Autodesk Inventor part; units mm, degrees
ref_plane "Work Plane1" through (8.89, -49.6518, 0) normal (1, 0, 0) x (0, 1, 0)
ref_plane "XZ Plane" through (0, 0, 0) normal (0, 1, 0) x (-1, 0, 0)
ref_plane "XY Plane" through (0, 0, 0) normal (0, 0, 1) x (1, 0, 0)
sketch "Sketch1" plane through (0, 0, 0) normal (0, 0, 1) x (1, 0, 0)
  line L0 (0, 0) -> (4.826, 4.3221)
  line L1 (4.826, 4.3221) -> (10.16, 0)
  line L2 (10.16, 0) -> (11.43, 6.2217)
  line L3 (0, 0) -> (-4.975, 5.229)
  arc A0 (11.43, 6.2217) -> (-4.975, 5.229) centre (5.08, -24.8868) ccw
  circle A1 centre (5.08, -24.8868) radius 25.4 construction
  circle A2 centre (5.08, -24.8868) radius 21.59 construction
  arc A3 (5.08, -47.1118) -> (7.7653, -46.949) centre (5.08, -24.8868) ccw
  circle A4 centre (5.08, -49.6518) radius 1.5875
  line L4 (5.08, -49.6518) -> (5.08, -46.4768) construction
  arc A5 (-14.879, -4.4376) -> (5.08, -53.4618) centre (5.08, -24.8868) ccw
  arc A6 (5.08, -53.4618) -> (7.7653, -46.949) centre (5.08, -49.6518) ccw
  line L5 (0, 0) -> (0, -3.2502)
  line L6 (-4.975, 5.229) -> (-14.879, -4.4376)
  arc A7 (0, -3.2502) -> (5.08, -47.1118) centre (5.08, -24.8868) ccw
  dimension "d40" = 43.18
  dimension "d0" = 31.75
  dimension "d2" = 50.8
  dimension "d3" = 29.21
  dimension "d4" = 30
  dimension "d5" = 10.16
  dimension "d6" = 5.334
  dimension "d42" = 44.45
  dimension "d43" = 3.175
  dimension "d44" = 3.175
  dimension "d47" = 3.81
extrude "Extrusion1" add sketch "Sketch1" along normal blind 6.35 contours L5 A7 A3 A6 A5 L6 L3
ref_plane "Work Plane1" through (8.89, -49.6518, 0) normal (1, 0, 0) x (0, 1, 0)
sketch "Sketch5" plane through (8.89, -49.6518, 0) normal (1, 0, 0) x (0, 1, 0)
  line L0 (-1.5875, 6.35) -> (1.5875, 6.35) construction
  line L1 (1.5875, 0) -> (-1.5875, 0) construction
  line L2 (-3.556, 1.397) -> (3.556, 1.397)
  line L3 (3.556, 1.397) -> (3.556, 4.953)
  line L4 (3.556, 4.953) -> (-3.556, 4.953)
  line L5 (-3.556, 4.953) -> (-3.556, 1.397)
  line L6 (-3.81, 0) -> (-3.81, 6.35) construction
  point P0 (49.6518, 0)
  point P1 (3.556, 3.175)
  point P2 (-3.81, 3.175)
  point P3 (0, 4.953)
  point P4 (0, 6.35)
  dimension "d48" = 3.556
  dimension "d49" = 7.112
extrude "Extrusion5" cut sketch "Sketch5" against normal blind 7.62
fillet "Fillet2" radius 1.27 5 edges at (7.7653, -46.949, 5.6515) (7.7653, -46.949, 0.6985) (0, -3.2502, 3.175) (0, 0, 3.175) (-4.975, 5.229, 3.175)
properties part number "BearingHolder1" material "ABS Plastic"
Input: part model. Units: mm. Frame: model coordinates. A direction names the side the tool comes from. Coordinates: 2 decimals unless noted, no trailing zeros. Loops run counter-clockwise (first coordinate to the right, second up) from the corner with the lowest first, then second, coordinate; pieces in that order, holes last. Notation, with made-up numbers: (-21, 45.25) - (16, 45.25) arc R16 cw to (16, 64.25) - close; hole circle Ø4 at (-11.75, -25.5). An arc over 180 degrees is marked (long way). Answer in a Markdown table with one row per item. Add a question column.
Item 1: Access query for faces 4 (the cylindrical face through (4.74, -48.1, 5.64)), 5 (the cylindrical face through (-0.265, -3.043, 3.219)), 6 (the cylindrical face through (6.108, -47.088, 5.642)), 7 (the flat face through (5.1, -51.4, 4.953)), 8 (the flat face through (0, -1, 3)). Directions: +Z, -Z, +X, -X, +Y, -Y. A direction counts if a zero-diameter tool reaches every point of the face in a straight line with its end or side. Return the directions, or none.
Item 2: Mould query, pull axis X, two halves, no side actions, for faces 1 (the cylindrical face through (7.93, -52.18, 5.25)), 2 (the cylindrical face through (4.74, -48.1, 0.69)), 3 (the flat face through (-17, -31, 6.35)). Classes: released by +X, released by -X, zero draft, split by the parting line, or undercut.
Item 3: Line query: line 1 along Y through (x, z) = (5.08, 5.8); line 2 along Y through (x, z) = (-9.5, 4); line 3 along X through (y, z) = (-49, 5). Output: solid intervals per line, ascending. Write a range as [from, to].
Item 4: Section query A-A on z = 2.25. Return the cut outline in (x, y) (3 decimals), then the cut area to 3 significant figures.
Item 5: Section query D-D on y = -14.5. Return the cut outline in (x, z).
Item 6: Section query C-C on x = -13. Return the cut outline in (y, z).
Item 7: Section query B-B on x = -8. Return the cut outline in (y, z).
Item 8: Contact query for flat-ended pins moving along their axis: P1, Ø5, axis at x = 5.5, y = -51, coming from the -Z side; P2, Ø1.4, axis at y = -1.5, z = 4, coming from the +X side; P3, Ø3, axis at y = -36, z = 3.5, coming from the -X side; P4, Ø1, axis at y = -40, z = 4, coming from the +X side. Output: stop coordinate, or through.
Recorded:
| question | item | result |
|---|---|---|
| 1 | face 4 | +Z, -Z |
| 1 | face 5 | +Z, -Z, +X |
| 1 | face 6 | +Z, -Z, +Y |
| 1 | face 7 | +X, +Y |
| 1 | face 8 | +Z, -Z, +X, +Y |
| 2 | face 1 | released by +X |
| 2 | face 2 | undercut |
| 2 | face 3 | zero draft |
| 3 | line 1 | [-53.46, -51.24], [-48.06, -47.11] |
| 3 | line 2 | [-49.46, -41.66], [-8.11, 0.81] |
| 3 | line 3 | [-10.25, 3.63], [6.53, 8.83] |
| 4 | outline | (-14.879, -4.438) arc R28.575 ccw to (1.27, -53.207) - (1.27, -46.783) arc R22.225 cw to (-0.927, -3.489) arc R1.27 ccw to (0, -2.266) - (0, -0.508) arc R1.27 ccw to (-0.35, 0.368) - (-4.088, 4.297) arc R1.27 ccw to (-5.896, 4.331) - close; (1.278, -53.208) arc R28.575 ccw to (5.08, -53.462) arc R3.81 ccw to (6.448, -53.208) - close |
| 4 | area | 462 mm^2 |
| 5 | outline | (-21.54, 0) - (-14.57, 0) - (-14.57, 6.35) - (-21.54, 6.35) - close |
| 6 | outline | (-47.01, 0) - (-37.81, 0) - (-37.81, 6.35) - (-47.01, 6.35) - close; (-11.96, 0) - (-2.6, 0) - (-2.6, 6.35) - (-11.96, 6.35) - close |
| 7 | outline | (-50.29, 0) - (-42.86, 0) - (-42.86, 6.35) - (-50.29, 6.35) - close; (-6.92, 0) - (2.28, 0) - (2.28, 6.35) - (-6.92, 6.35) - close |
| 8 | P1 | z = 0 |
| 8 | P2 | x = 0 |
| 8 | P3 | x = -21.83 |
| 8 | P4 | x = -10.74 |
